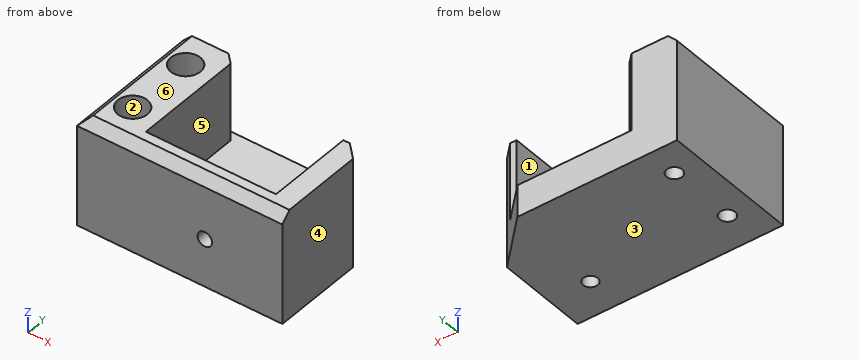
```python
from build123d import *

# Parameters (mm, degrees)
SKETCH_1_W                  = 45
SKETCH_1_H                  = 30
EXTRUDE_1_DEPTH             = 24
SKETCH_2_W                  = 17
SKETCH_2_H                  = 6.914213562
CUT_EXTRUDE_1_DEPTH         = 33
CUT_EXTRUDE_2_REACH         = 62.975
SKETCH_4_W                  = 28.5
SKETCH_4_H                  = 17
HOLE_WIZARD_3_2_3_2_1_D     = 3.2
HOLE_WIZARD_3_2_3_2_2_D     = 3.2
HOLE_WIZARD_M31_D           = 3.4
HOLE_WIZARD_M31_CBORE_D     = 6.5
HOLE_WIZARD_M31_CBORE_DEPTH = 15
CHAMFER_1_SIZE              = 2
CHAMFER_2_SIZE              = 10


with BuildPart() as part:
    # Эскиз1 → Бобышка-Вытянуть1 (new body)
    with BuildSketch(Plane.XY.offset(21)):
        with Locations((28.500002027, 21)):
            Rectangle(SKETCH_1_W, SKETCH_1_H)
    extrude(amount=-EXTRUDE_1_DEPTH)

    # Эскиз2 → Вырез-Вытянуть1 (cut)
    with BuildSketch(Plane(origin=(51.000002027, 0, 0), x_dir=(0, 0, -1), z_dir=(1, 0, 0))):
        with Locations((-12.5, 32.542893219)):
            Rectangle(SKETCH_2_W, SKETCH_2_H)
    extrude(amount=-CUT_EXTRUDE_1_DEPTH, mode=Mode.SUBTRACT)

    # Эскиз4 → Вырез-Вытянуть2 (cut, up to next)
    with BuildSketch(Plane.XZ.offset(-10), mode=Mode.PRIVATE) as cut_extrude_2_sk1:
        with Locations((32.250002027, 12.5)):
            Rectangle(SKETCH_4_W, SKETCH_4_H)
    cut_extrude_2_tool1 = extrude(cut_extrude_2_sk1.sketch, amount=-CUT_EXTRUDE_2_REACH, mode=Mode.PRIVATE) & part.part
    add(cut_extrude_2_tool1.solids().sort_by_distance((32.250002, 10, 12.5))[0], mode=Mode.SUBTRACT)

    # Диаметр отверстия Ø3.2 (3.2)1 (through all)
    with Locations(Plane.XY.offset(4)):
        with Locations((42.000002027, 14)):
            Hole(HOLE_WIZARD_3_2_3_2_1_D / 2)

    # Диаметр отверстия Ø3.2 (3.2)2 (through all)
    with Locations(Plane(origin=(0, 10, 0), x_dir=(1, 0, 0), z_dir=(0, 1, 0))):
        with Locations((34.000002027, -7.5)):
            Hole(HOLE_WIZARD_3_2_3_2_2_D / 2)

    # Цековка для винта с заклепочной головкой M31 (through all)
    with Locations(Plane.XY.offset(21)):
        with Locations((12.000002027, 29), (12.000002027, 14)):
            CounterBoreHole(HOLE_WIZARD_M31_D / 2, HOLE_WIZARD_M31_CBORE_D / 2, HOLE_WIZARD_M31_CBORE_DEPTH)

    # Фаска1
    chamfer_1_edges = [part.edges().sort_by_distance(p)[0] for p in [
        (18.000002027, 36, 12.5),
        (6.000002027, 21, 21),
        (28.500002027, 6, 21),
    ]]
    chamfer(chamfer_1_edges, length=CHAMFER_1_SIZE)

    # Фаска2
    chamfer_2_edges = [part.edges().sort_by_distance(p)[0] for p in [
        (51.000002027, 36, 0.5),
    ]]
    chamfer(chamfer_2_edges, length=CHAMFER_2_SIZE)


solid = part.part
```
Model file for the job. Use its own axes, mm. Face numbers are marked on the shaded views. A direction names the side the tool comes from. Give positions to 0.01 mm unless a question says otherwise; leave off trailing zeros. Write each loop counter-clockwise with the first axis right and the second up, starting at its lowest first coordinate (ties: lowest second). Pieces come first, ordered by that corner, then holes. Notation, with made-up numbers: (4, 73.5) - (53, 73.5) arc R29 ccw to (53, 98.5) - close; hole circle Ø11 at (18, 20.25). An arc over 180 degrees is marked (long way). One line per question, with ' | ' between items. Start each with the question number.
(1) Two-plate mould, pull along X, no slides. Class the marked faces 4, 5 and 6: +X half, -X half, draft (parallel to the pull), parting line (faces both ways), or undercut.
(2) 3-axis set-ups, long thin cutter, end or side, ignore diameter. For the marked faces 1, 2 and 3: which of +Z, -Z, +X, -X, +Y, -Y reach the whole face in a straight line?
(3) Wall check: line 1 along Y through (x, z) = (15, 12); line 2 along Y through (x, z) = (11, 9.25); line 3 along X through (y, z) = (22.5, 9). Give the ranges that are in metal, low to high. Write a range as from..to.
(4) Pin check, flat tips, straight feed: P1, Ø3.5, axis at x = 42, y = 14, coming from the +Z side; P2, Ø2, axis at x = 10.5, y = 13.5, coming from the +Z side; P3, Ø1.9, axis at x = 34, z = 7.5, coming from the -Y side; P4, Ø1.6, axis at x = 47, z = 8.5, coming from the +Y side. Stop position of each tip, or through.
(5) Slice it at A-A on z = 7.5. Write the cut outline in (x, y), plus the area to 3 significant figures.
(6) Slice it at D-D on x = 38.5. Write the cut outline in (y, z).
(7) Slice it at B-B on z = 18.25. Write the cut outline in (x, y).
(8) Slice it at C-C on y = 14. Write the cut outline in (x, z), plus the area to 3 significant figures.
Results below:
1) face 4: +X half | face 5: undercut | face 6: draft
2) face 1: +Z, +Y | face 2: +Z | face 3: -Z, +X, -X, +Y, -Y
3) line 1: 6..12.75, 15.25..27.75, 30.25..36 | line 2: 6..10.91, 17.09..25.91, 32.09..36 | line 3: 6..18, 46.5..51
4) P1: z = 4 | P2: z = 6 | P3: through | P4: y = 29.09
5) outline: (6, 6) - (32.4, 6) - (32.4, 10) - (18, 10) - (18, 34) - (16, 36) - (6, 36) - close; (35.6, 6) - (51, 6) - (51, 26) - (47.91, 29.09) - (46.5, 29.09) - (46.5, 10) - (35.6, 10) - close; hole circle Ø6.5 at (12, 14); hole circle Ø6.5 at (12, 29) | area: 492 mm^2
6) outline: (6, -3) - (36, -3) - (36, 4) - (10, 4) - (10, 21) - (8, 21) - (6, 19) - close
7) outline: (6, 6) - (51, 6) - (51, 26) - (47.91, 29.09) - (46.5, 29.09) - (46.5, 10) - (18, 10) - (18, 34) - (16, 36) - (6, 36) - close; hole circle Ø6.5 at (12, 14); hole circle Ø6.5 at (12, 29)
8) outline: (6, -3) - (10.3, -3) - (10.3, 6) - (8.75, 6) - (8.75, 21) - (8, 21) - (6, 19) - close; (13.7, -3) - (40.4, -3) - (40.4, 4) - (18, 4) - (18, 21) - (15.25, 21) - (15.25, 6) - (13.7, 6) - close; (43.6, -3) - (51, -3) - (51, 21) - (46.5, 21) - (46.5, 4) - (43.6, 4) - close | area: 443 mm^2
